Part model, mm, in its own coordinate system. Face numbers are marked on the shaded views. Round coordinates to 2 decimals unless told otherwise and drop trailing zeros. Answer as a JSON object with one key per item and string values. Group by question number.
1. Two-plate mould, pull along X, no slides. Class the marked faces 1, 2 and 3: +X half, -X half, draft (parallel to the pull), parting line (faces both ways), or undercut.
2. Drop flat-ended pins along their axis: pin 1 (2 mm diameter, centred on x = 44.5, z = -21.5, fed in from +Y); pin 2 (10 mm diameter, centred on x = 50, z = 43, fed in from +Y); pin 3 (8 mm diameter, centred on x = -15.5, y = -16, fed in from +Z). Give the stop position or say it passes through.
3. Drill centre lines: line 1 (Y direction, x = -35, z = -1.5); line 2 (Z direction, x = 30.5, y = -3.75); line 3 (X direction, y = -11.5, z = 14). Where is each one in solid material? Low to high. Write a range as from..to.
from build123d import *

# Parameters (mm, degrees)
SKETCH1_R           = 100
BOSS_EXTRUDE1_DEPTH = 10
BOSS_EXTRUDE1_DRAFT = -60
SKETCH2_R           = 82.679491924
BOSS_EXTRUDE2_DEPTH = 10
BOSS_EXTRUDE2_TAPER = 40
FILLET1_R           = 10
FILLET2_R           = 2


# Read off the part's stored shape, not the designer's step: Shell2
with BuildPart() as part:
    # Sketch1 → Boss-Extrude1 (with draft: the straight prism first)
    with BuildSketch(Plane(origin=(0, 0, 0), x_dir=(1, 0, 0), z_dir=(0, 1, 0))):
        Circle(SKETCH1_R)
    extrude(amount=-BOSS_EXTRUDE1_DEPTH)
    # Boss-Extrude1: the draft: its side faces are tilted about the plane it starts from
    boss_extrude1_sides = [part.faces().sort_by_distance(p)[0] for p in [
        (-100, -5, 0),
    ]]
    draft(boss_extrude1_sides, Plane(origin=(0, 0, 0), x_dir=(1, 0, 0), z_dir=(0, 1, 0)), BOSS_EXTRUDE1_DRAFT)

    # Sketch2 → Boss-Extrude2 (add)
    with BuildSketch(Plane.XZ.offset(10)):
        Circle(SKETCH2_R)
    extrude(amount=BOSS_EXTRUDE2_DEPTH, taper=BOSS_EXTRUDE2_TAPER)

    # Fillet1
    fillet1_edges = [part.edges().sort_by_distance(p)[0] for p in [
        (-82.679491924, -10, 0),
        (-74.288495613, -20, 0),
    ]]
    fillet(fillet1_edges, radius=FILLET1_R)

    # Fillet2
    fillet2_edges = [part.edges().sort_by_distance(p)[0] for p in [
        (-100, 0, 0),
    ]]
    fillet(fillet2_edges, radius=FILLET2_R)

    # Shell2 outline → Shell2 (revolve, cut)
    with BuildSketch(Plane.XY):
        with BuildLine():
            ThreePointArc((77.715861724, -8.136804989), (79.564714226, -6.287952488), (81.706528371, -4.788238078))
            Line((81.706528371, -4.788238078), (90, 0))
            Line((90, 0), (0, 0))
            Line((0, 0), (0, -15))
            Line((0, -15), (69.625419031, -15))
            ThreePointArc((69.625419031, -15), (71.73851034, -14.531538935), (73.455641247, -13.213938048))
            Line((73.455641247, -13.213938048), (77.715861724, -8.136804989))
        make_face()
    revolve(axis=Axis((0, 0, 0), (0, 1, 0)), mode=Mode.SUBTRACT)


solid = part.part
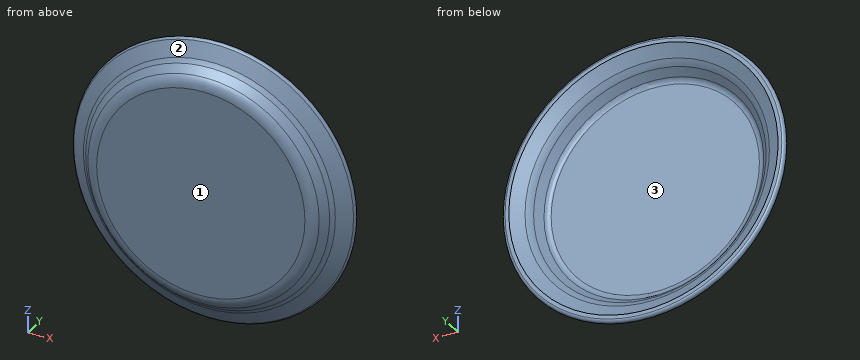
Worked answers:
{
 "1": {"face 1": "draft", "face 2": "parting line", "face 3": "undercut"},
 "2": {"pin 1": "stops at y = -15", "pin 2": "stops at y = -14.82", "pin 3": "stops at z = 79.59"},
 "3": {"line 1": "y = -20..-15", "line 2": "z = -88.39..-77.74, 77.74..88.39", "line 3": "x = -80.21..-73.57, 73.57..80.21"}
}
